Part model, mm, in its own coordinate system. A direction names the side the tool comes from. Coordinates: 2 decimals unless noted, no trailing zeros. Order: outer loops, then holes, each group sorted by start corner. A loop starts at its lowest first (then second) coordinate and runs counter-clockwise, first axis right, second up.
1) Cut at B-B (y = 9.25). List the corners of the cut face in (x, z), and give its area (3 significant figures).
2) Pin check, flat tips, straight feed: pin 1 Ø4 at (x, y) = (-8, -4.5) entering from +Z; pin 2 Ø10 at (x, y) = (4.5, -9) entering from +Z; pin 3 Ø3.5 at (x, y) = (0, -0.5) entering from +Z. Stop position of each tip, or through.
3) Cut at C-C (z = 2.5). Give the number of separate pieces and of enclosed holes in the cut face, and give its area (3 significant figures).
4) Wall check: L1, parallel to X at y = 0, z = 6 (3 decimals); L2, parallel to X at y = 3, z = 1.25; L3, parallel to Y at x = -9.75, z = 4.75. Give the ranges that are in metal, low to high.
5) Tool access for faces 1 (the flat face through (15, 0, 4)), 2 (the flat face through (0, -13, 5)): list every direction of +Z, -Z, +X, -X, +Y, -Y with a clear straight run to the whole face (end or side of a thin tool).
6) Cut at A-A (z = 9). List the corners of the cut face in (x, y), and give its area (3 significant figures).
```python
from build123d import *

# Parameters (mm, degrees)
EXTRUDE_1_DEPTH = 10
EXTRUDE_2_DEPTH = 8
EXTRUDE_START   = -2
EXTRUDE_3_DEPTH = 2
EXTRUDE_4_DEPTH = 2


with BuildPart() as part:
    # Sketch 1 → Extrude 1 (new body)
    with BuildSketch(Plane.XY):
        with BuildLine():
            ThreePointArc((-15, 13), (-14.414213562, 14.414213562), (-13, 15))
            Line((-13, 15), (13, 15))
            ThreePointArc((13, 15), (14.414213562, 14.414213562), (15, 13))
            Line((15, 13), (15, -13))
            ThreePointArc((15, -13), (14.414213562, -14.414213562), (13, -15))
            Line((13, -15), (-13, -15))
            ThreePointArc((-13, -15), (-14.414213562, -14.414213562), (-15, -13))
            Line((-15, -13), (-15, 13))
        make_face()
        with BuildLine():
            ThreePointArc((-13, -11), (-12.414213562, -12.414213562), (-11, -13))
            Line((-11, -13), (11, -13))
            ThreePointArc((11, -13), (12.414213562, -12.414213562), (13, -11))
            Line((13, -11), (13, 11))
            ThreePointArc((13, 11), (12.414213562, 12.414213562), (11, 13))
            Line((11, 13), (-11, 13))
            ThreePointArc((-11, 13), (-12.414213562, 12.414213562), (-13, 11))
            Line((-13, 11), (-13, -11))
        make_face(mode=Mode.SUBTRACT)
    extrude(amount=EXTRUDE_1_DEPTH)



with BuildPart() as body_2:
    # Sketch 1_6 → Extrude 2 (new body)
    with BuildSketch(Plane.XY):
        with BuildLine():
            ThreePointArc((0.25, 2.788816953), (0, 2.8), (-0.25, 2.788816953))
            ThreePointArc((-0.25, 2.788816953), (-1.979898987, 1.979898987), (-2.788816953, 0.25))
            ThreePointArc((-2.788816953, 0.25), (-2.8, 0), (-2.788816953, -0.25))
            ThreePointArc((-2.788816953, -0.25), (-1.979898987, -1.979898987), (-0.25, -2.788816953))
            ThreePointArc((-0.25, -2.788816953), (0, -2.8), (0.25, -2.788816953))
            ThreePointArc((0.25, -2.788816953), (1.979898987, -1.979898987), (2.788816953, -0.25))
            ThreePointArc((2.788816953, -0.25), (2.797202841, -0.125124998), (2.8, 0))
            ThreePointArc((2.8, 0), (2.797202841, 0.125124998), (2.788816953, 0.25))
            ThreePointArc((2.788816953, 0.25), (1.979898987, 1.979898987), (0.25, 2.788816953))
        make_face()
        Polygon((-2.175, -0.7), (-2.175, 0.7), (-0.7, 0.7), (-0.7, 2.175), (0.7, 2.175), (0.7, 0.7), (2.175, 0.7), (2.175, -0.7), (0.7, -0.7), (0.7, -2.175), (-0.7, -2.175), (-0.7, -0.7), align=None, mode=Mode.SUBTRACT)
    extrude(amount=EXTRUDE_2_DEPTH)


with BuildPart() as part_1:
    add(part.part)

    add(body_2.part)  # Extrude 3 merges body 2
    # Sketch 1_7 → Extrude 3 (add)
    with BuildSketch(Plane.XY.offset(EXTRUDE_START)):
        with BuildLine():
            Line((-13, 15), (13, 15))
            ThreePointArc((13, 15), (14.414213562, 14.414213562), (15, 13))
            Line((15, 13), (15, -13))
            ThreePointArc((15, -13), (14.414213562, -14.414213562), (13, -15))
            Line((13, -15), (-13, -15))
            ThreePointArc((-13, -15), (-14.414213562, -14.414213562), (-15, -13))
            Line((-15, -13), (-15, 13))
            ThreePointArc((-15, 13), (-14.414213562, 14.414213562), (-13, 15))
        make_face()
    extrude(amount=EXTRUDE_3_DEPTH)

    # Sketch 1_9 → Extrude 4 (add)
    with BuildSketch(Plane.XY):
        with BuildLine():
            Line((-2.788816953, 0.25), (-13, 0.25))
            Line((-13, 0.25), (-13, -0.25))
            Line((-13, -0.25), (-2.788816953, -0.25))
            ThreePointArc((-2.788816953, -0.25), (-2.8, 0), (-2.788816953, 0.25))
        make_face()
        with BuildLine():
            Line((0.25, 13), (-0.25, 13))
            Line((-0.25, 13), (-0.25, 2.788816953))
            ThreePointArc((-0.25, 2.788816953), (0, 2.8), (0.25, 2.788816953))
            Line((0.25, 2.788816953), (0.25, 13))
        make_face()
        with BuildLine():
            Line((13, 0.25), (2.788816953, 0.25))
            ThreePointArc((2.788816953, 0.25), (2.797202841, 0.125124998), (2.8, 0))
            ThreePointArc((2.8, 0), (2.797202841, -0.125124998), (2.788816953, -0.25))
            Line((2.788816953, -0.25), (13, -0.25))
            Line((13, -0.25), (13, 0.25))
        make_face()
        with BuildLine():
            ThreePointArc((0.25, -2.788816953), (0, -2.8), (-0.25, -2.788816953))
            Line((-0.25, -2.788816953), (-0.25, -13))
            Line((-0.25, -13), (0.25, -13))
            Line((0.25, -13), (0.25, -2.788816953))
        make_face()
    extrude(amount=EXTRUDE_4_DEPTH)


solid = part_1.part
```
Geometry check:
1. outline: (-15, -2) - (15, -2) - (15, 10) - (13, 10) - (13, 0) - (0.25, 0) - (0.25, 2) - (-0.25, 2) - (-0.25, 0) - (-13, 0) - (-13, 10) - (-15, 10) - close
1. area: 101 mm2
2. pin 1: stops at z = 0
2. pin 2: stops at z = 10
2. pin 3: stops at z = 8
3. separate pieces: 2
3. enclosed holes: 2
3. area: 238 mm2
4. L1: x = -15 to -13, -2.8 to -2.175, 2.175 to 2.8, 13 to 15
4. L2: x = -15 to -13, -0.25 to 0.25, 13 to 15
4. L3: y = -15 to -13, 13 to 15
5. face 1: +Z, -Z, +X, +Y, -Y
5. face 2: +Z
6. outline: (-15, -13) arc R2 ccw to (-13, -15) - (13, -15) arc R2 ccw to (15, -13) - (15, 13) arc R2 ccw to (13, 15) - (-13, 15) arc R2 ccw to (-15, 13) - close; hole (-13, -11) arc R2 ccw to (-11, -13) - (11, -13) arc R2 ccw to (13, -11) - (13, 11) arc R2 ccw to (11, 13) - (-11, 13) arc R2 ccw to (-13, 11) - close
6. area: 224 mm2
